Read the model definition and answer for the solid it produces. Units are mm, in the model's axes. Give positions to 0.01 mm unless a question says otherwise; leave off trailing zeros. Write each loop counter-clockwise with the first axis right and the second up, starting at its lowest first coordinate (ties: lowest second). Pieces come first, ordered by that corner, then holes.
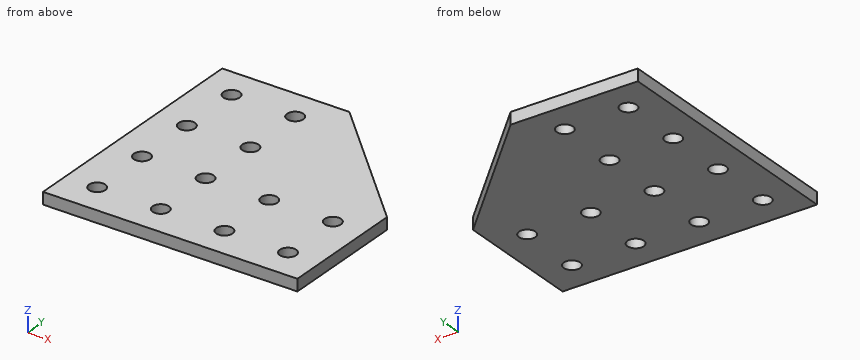
```python
from build123d import *

# Parameters (mm, degrees)
SKETCH1_R           = 3.2639
BOSS_EXTRUDE1_DEPTH = 2.38125


with BuildPart() as part:
    # Sketch1 → Boss-Extrude1 (new body, symmetric)
    with BuildSketch(Plane.XY):
        Polygon((0, 0), (0, 101.6), (50.8, 101.6), (101.6, 50.8), (101.6, 0), align=None)
        with Locations((12.7, 12.7)):
            Circle(SKETCH1_R, mode=Mode.SUBTRACT)
        with Locations((38.1, 12.7)):
            Circle(SKETCH1_R, mode=Mode.SUBTRACT)
        with Locations((63.5, 12.7)):
            Circle(SKETCH1_R, mode=Mode.SUBTRACT)
        with Locations((12.7, 38.1)):
            Circle(SKETCH1_R, mode=Mode.SUBTRACT)
        with Locations((12.7, 63.5)):
            Circle(SKETCH1_R, mode=Mode.SUBTRACT)
        with Locations((88.9, 12.7)):
            Circle(SKETCH1_R, mode=Mode.SUBTRACT)
        with Locations((88.9, 38.1)):
            Circle(SKETCH1_R, mode=Mode.SUBTRACT)
        with Locations((63.5, 38.1)):
            Circle(SKETCH1_R, mode=Mode.SUBTRACT)
        with Locations((38.1, 38.1)):
            Circle(SKETCH1_R, mode=Mode.SUBTRACT)
        with Locations((12.7, 88.9)):
            Circle(SKETCH1_R, mode=Mode.SUBTRACT)
        with Locations((38.1, 88.9)):
            Circle(SKETCH1_R, mode=Mode.SUBTRACT)
        with Locations((38.1, 63.5)):
            Circle(SKETCH1_R, mode=Mode.SUBTRACT)
    extrude(amount=BOSS_EXTRUDE1_DEPTH, both=True)


solid = part.part
```
Item 1: Find the intervals of material crossed by line 1 along X through (y, z) = (12.5, -0.8); line 2 along X through (y, z) = (40, -1.4); line 3 along X through (y, z) = (61.5, 0.55), in increasing order.
Result set:
line 1: x = 0 to 9.44, 15.96 to 34.84, 41.36 to 60.24, 66.76 to 85.64, 92.16 to 101.6
line 2: x = 0 to 10.05, 15.35 to 35.45, 40.75 to 60.85, 66.15 to 86.25, 91.55 to 101.6
line 3: x = 0 to 10.12, 15.28 to 35.52, 40.68 to 90.9
Item 2: Section C-C (y = 63.5) is taken. Write down the section's boundary in (x, z), and give its area (3 significant figures).
Result set:
outline: (0, -2.38) - (9.44, -2.38) - (9.44, 2.38) - (0, 2.38) - close; (15.96, -2.38) - (34.84, -2.38) - (34.84, 2.38) - (15.96, 2.38) - close; (41.36, -2.38) - (88.9, -2.38) - (88.9, 2.38) - (41.36, 2.38) - close
area: 361 mm2
Item 3: Section A-A (y = 12.7) is taken. Write down the section's boundary in (x, z), and give its area (3 significant figures).
Result set:
outline: (0, -2.38) - (9.44, -2.38) - (9.44, 2.38) - (0, 2.38) - close; (15.96, -2.38) - (34.84, -2.38) - (34.84, 2.38) - (15.96, 2.38) - close; (41.36, -2.38) - (60.24, -2.38) - (60.24, 2.38) - (41.36, 2.38) - close; (66.76, -2.38) - (85.64, -2.38) - (85.64, 2.38) - (66.76, 2.38) - close; (92.16, -2.38) - (101.6, -2.38) - (101.6, 2.38) - (92.16, 2.38) - close
area: 360 mm2
Item 4: Each of these flat-tipped pins is pushed along its axis until it touches: pin 1 Ø6 at (x, y) = (88.9, 38.1) entering from -Z; pin 2 Ø1.5 at (y, z) = (75.5, 0) entering from +X. Where does it stop, or does it pass through?
Result set:
pin 1: passes through
pin 2: stops at x = 77.65
